Geometry: final body of the model. Coordinates: model frame, mm. A direction names the side the tool comes from. Round coordinates to 2 decimals unless told otherwise and drop trailing zeros. Write each loop counter-clockwise with the first axis right and the second up, starting at its lowest first coordinate (ties: lowest second). Pieces come first, ordered by that corner, then holes. Notation, with made-up numbers: M 57.5,11.25 L 64.5,11.25 A14 ccw 64.5,25.25 Z; hole C 78,89.25 d10. An arc over 180 degrees is marked long. Use one line per item in the form item = value. Start each with the question number.
from build123d import *

# Parameters (mm, degrees)
SKETCH1_W                         = 2
SKETCH1_H                         = 40
BULK_EXTRUDE_ANGLE                = 20
CONNECTOR_PASSTHRU_DEPTH          = 41.516317865
CONNECTOR_PASSTHRU_DEPTH_BACK     = 41.516317865
SKETCH2_R                         = 1.25
SKETCH2_W                         = 9.4
SKETCH2_H                         = 27.2
REAR_FLATTENING_REACH             = 42.516
SKETCH3_W                         = 11.20030746
SKETCH3_H                         = 40
SKETCH3_R                         = 1.25
SKETCH3_W_2                       = 9.4
SKETCH3_H_2                       = 27.2
REAR_FLATTENING_DIRECTION_2_DEPTH = 1.5
SKETCH4_W                         = 5.422124609
SKETCH4_H                         = 40
CUT_EXTRUDE2_DEPTH                = 42.810193065
SKETCH5_W                         = 5.376196321
SKETCH5_H                         = 40
CUT_EXTRUDE3_DEPTH                = 42.810193065
FILLET1_R                         = 3


with BuildPart() as part:
    # Sketch1 → BULK EXTRUDE (revolve, symmetric)
    with BuildSketch(Plane(origin=(0, 0, 0), x_dir=(0, 0, -1), z_dir=(1, 0, 0))) as bulk_extrude_sk:
        with Locations((1, 20)):
            Rectangle(SKETCH1_W, SKETCH1_H)
    revolve(axis=Axis((0, 0, -34.25), (0, 1, 0)), revolution_arc=BULK_EXTRUDE_ANGLE / 2)
    revolve(bulk_extrude_sk.sketch, axis=Axis((0, 0, -34.25), (0, -1, 0)), revolution_arc=BULK_EXTRUDE_ANGLE / 2)

    # Sketch2 → CONNECTOR PASSTHRU (cut, two sides: drawn at the far end of the back side and taken through both)
    with BuildSketch(Plane.XY.offset(-CONNECTOR_PASSTHRU_DEPTH_BACK)):
        with Locations((0, 4.52)):
            Circle(SKETCH2_R)
        with Locations((0, 35.48)):
            Circle(SKETCH2_R)
        with Locations((0, 20)):
            Rectangle(SKETCH2_W, SKETCH2_H)
    extrude(amount=CONNECTOR_PASSTHRU_DEPTH + CONNECTOR_PASSTHRU_DEPTH_BACK, mode=Mode.SUBTRACT)

    # Sketch3 → REAR FLATTENING (add, up to next)
    with BuildSketch(Plane.XY.offset(-2.489949965), mode=Mode.PRIVATE) as rear_flattening_sk1:
        with Locations((0, 20)):
            Rectangle(SKETCH3_W, SKETCH3_H)
        with Locations((0, 4.52)):
            Circle(SKETCH3_R, mode=Mode.SUBTRACT)
        with Locations((0, 35.48)):
            Circle(SKETCH3_R, mode=Mode.SUBTRACT)
        with Locations((0, 20)):
            Rectangle(SKETCH3_W_2, SKETCH3_H_2, mode=Mode.SUBTRACT)
    rear_flattening_tool1 = extrude(rear_flattening_sk1.sketch, amount=REAR_FLATTENING_REACH, mode=Mode.PRIVATE) - part.part
    add(rear_flattening_tool1.solids().sort_by_distance((0, 0.415385, -2.48995))[0])

    # Sketch3 → REAR FLATTENING direction 2 (add)
    with BuildSketch(Plane.XY.offset(-2.489949965)):
        with Locations((0, 20)):
            Rectangle(SKETCH3_W, SKETCH3_H)
        with Locations((0, 4.52)):
            Circle(SKETCH3_R, mode=Mode.SUBTRACT)
        with Locations((0, 35.48)):
            Circle(SKETCH3_R, mode=Mode.SUBTRACT)
        with Locations((0, 20)):
            Rectangle(SKETCH3_W_2, SKETCH3_H_2, mode=Mode.SUBTRACT)
    extrude(amount=-REAR_FLATTENING_DIRECTION_2_DEPTH)

    # Sketch4 → Cut-Extrude2 (cut, through all)
    with BuildSketch(Plane(origin=(5.857094954, 0, -1.032763869), x_dir=(-0.17364817766693075, 0, -0.9848077530122081), z_dir=(0.9848077530122081, 0, -0.17364817766693075))):
        with Locations((2.190727846, 20)):
            Rectangle(SKETCH4_W, SKETCH4_H)
    extrude(amount=CUT_EXTRUDE2_DEPTH, mode=Mode.SUBTRACT)

    # Sketch5 → Cut-Extrude3 (cut, through all)
    with BuildSketch(Plane(origin=(-5.857094954, 0, -1.032763869), x_dir=(-0.17364817766693072, 0, 0.9848077530122081), z_dir=(-0.9848077530122081, 0, -0.17364817766693072))):
        with Locations((-2.167763702, 20)):
            Rectangle(SKETCH5_W, SKETCH5_H)
    extrude(amount=CUT_EXTRUDE3_DEPTH, mode=Mode.SUBTRACT)

    # Fillet1
    fillet1_edges = [part.edges().sort_by_distance(p)[0] for p in [
        (5.641556672, 40, -2.255142212),
        (-5.641556672, 0, -2.255142212),
        (-5.641556672, 40, -2.255142212),
        (5.641556672, 0, -2.255142212),
    ]]
    fillet(fillet1_edges, radius=FILLET1_R)

    # Sketch6 → Cut-Revolve1 (revolve, cut)
    with BuildSketch(Plane.ZY, mode=Mode.PRIVATE) as cut_revolve1_sk:
        Polygon((0, 4.52), (0, 6.27), (-1, 5.645), (-1, 4.52), align=None)
    cut_revolve1 = revolve(cut_revolve1_sk.sketch.rotate(Axis((0, 4.52, -3.989949965), (0, 0, 1)), 270), axis=Axis((0, 4.52, -3.989949965), (0, 0, 1)), mode=Mode.SUBTRACT)

    # Mirror1: Cut-Revolve1 across plane
    add(cut_revolve1.mirror(Plane.ZX.offset(20)), mode=Mode.SUBTRACT)


solid = part.part
1. Section query B-B (y = 13.5). Return loops of the section in (x, z), then the cut area to 3 significant figures.
2. Set-up query: faces 1 (the face through (0, 0, -2)), 2 (the face through (0, 33.6, -2)). Return all of +Z, -Z, +X, -X, +Y, -Y with unobstructed straight access to the full face (end or side cutting, diameter ignored); none if empty.
3. Section query A-A (x = 0). Return loops of the section in (y, z).
4. Contact query for flat-ended pins moving along their axis: pin 1 (1 mm diameter, centred on x = 2, y = 34, fed in from +Z); pin 2 (1.1 mm diameter, centred on y = 14.5, z = -1.5, fed in from -X); pin 3 (5 mm diameter, centred on x = 2.5, y = 11.5, fed in from +Z). Output: stop coordinate, or through.
5. Section query C-C (y = 35.48). Return loops of the section in (x, z).
6. Pull-direction query (X, two-part tool) for faces 3 (the face through (0, 6.4, -2)), 4 (the face through (4.748, 0.902, -2.395)), 5 (the face through (-4.748, 0.902, -2.395)), 6 (the face through (5.375, 24.724, -0.424)); classes: released by +X, released by -X, zero draft, split by the parting line, or undercut.
7. Ray query, probe 1 along Y at (x, z) = (0, -1.4); probe 2 along Y at (x, z) = (2.25, -0.4); probe 3 along X at (y, z) = (12, -0.85). Return the intervals inside material, ascending.
Checks:
q1.outline = M -5.95,-0.52 L -5.34,-3.99 L -4.7,-3.99 L -4.7,-0.32 A34.25 ccw Z; M 4.7,-3.99 L 5.34,-3.99 L 5.95,-0.52 A34.25 ccw 4.7,-0.32 Z
q1.area = 6.79 mm^2
q2.face_1 = +Z, -Z, +X, -X, -Y
q2.face_2 = +Z, -Z
q3.outline = M 0,-3.99 L 3.27,-3.99 L 3.27,-0.8 L 2.77,0 L 0,0 Z; M 5.77,-3.99 L 6.4,-3.99 L 6.4,0 L 6.27,0 L 5.77,-0.8 Z; M 33.6,-3.99 L 34.23,-3.99 L 34.23,-0.8 L 33.73,0 L 33.6,0 Z; M 36.73,-3.99 L 40,-3.99 L 40,0 L 37.23,0 L 36.73,-0.8 Z
q4.pin_1 = -0.03
q4.pin_2 = -5.87
q4.pin_3 = -0.32
q5.outline = M -5.95,-0.52 L -5.34,-3.99 L -1.25,-3.99 L -1.25,-0.8 L -1.72,-0.04 A34.25 ccw Z; M 1.25,-3.99 L 5.34,-3.99 L 5.95,-0.52 A34.25 ccw 1.72,-0.04 L 1.25,-0.8 Z
q6.face_3 = undercut
q6.face_4 = released by +X
q6.face_5 = released by -X
q6.face_6 = split by the parting line
q7.probe_1 = 0 to 3.27, 5.77 to 6.4, 33.6 to 34.23, 36.73 to 40
q7.probe_2 = 0 to 6.4, 33.6 to 40
q7.probe_3 = -5.89 to -4.7, 4.7 to 5.89
